The listing builds one solid part. Answer for the finished solid, in the listing's coordinates (mm). Face numbers are marked on the shaded views. A direction names the side the tool comes from. Coordinates: 2 decimals unless noted, no trailing zeros. Write each loop counter-clockwise with the first axis right and the second up, starting at its lowest first coordinate (ties: lowest second). Pieces come first, ordered by that corner, then holes.
(1) The part is cut by section D-D on x = -23. Determine the outline of the cut face in (y, z).
(2) Given P1, Ø4, axis at y = -25.5, z = -17.5, coming from the -X side; P2, Ø6, axis at x = 50.5, y = 28, coming from the -Z side; P3, Ø5.5, axis at y = 29.5, z = -18, coming from the -X side, each flat-ended and moving along its own axis, determine where each tip first touches the part or whether it passes through.
(3) The part is cut by section B-B on z = 8.5. Determine the outline of the cut face in (x, y).
(4) The part is cut by section C-C on y = 0. Determine the outline of the cut face in (x, z).
(5) The part is cut by section A-A on x = -66.5. Determine the outline of the cut face in (y, z).
(6) For a pull along X with two mould halves and no side action, classify the marked faces 1, 2 and 3 as +X half, -X half, draft (parallel to the pull), parting line (faces both ways), or undercut.
(7) Straight lines are drawn through the part: line 1 (Y direction, x = -32, z = 2); line 2 (Y direction, x = 40.5, z = -1.5); line 3 (Z direction, x = -31, y = -15). For each, find the intervals that lie inside material, in ascending order.
(8) Which of the six approach directions +Z, -Z, +X, -X, +Y, -Y give full straight-line access (tool end or side, diameter ignored) to the marked faces 4 and 5?
from build123d import *

# Parameters (mm, degrees)
F0_W      = 208
F0_H      = 50
F1_DEPTH  = 37.5
F2_R      = 32.5
F3_DEPTH  = 50.001
F4_W      = 128
F4_H      = 65
F5_DEPTH  = 45
F6_W      = 65
F6_H      = 5
F7_DEPTH  = 5
F8_W      = 10
F8_H      = 10
F9_DEPTH  = 5
F10_R     = 2
F11_DEPTH = 9.8017221311
F12_R     = 32.5
F13_W     = 125
F13_H     = 5
F14_DEPTH = 8
F16_DEPTH = 75.001


with BuildPart() as f1:
    # F0 (on Front) → F1 (new body, symmetric)
    with BuildSketch(Plane.XZ):
        Rectangle(F0_W, F0_H)
    extrude(amount=F1_DEPTH, both=True)

    # F2 (on face) → F3 (cut, through all)
    with BuildSketch(Plane.XY.offset(25)):
        with Locations((-66.5, 0)):
            Circle(F2_R)
    extrude(amount=-F3_DEPTH, mode=Mode.SUBTRACT)

    # F4 (on face) → F5 (cut)
    with BuildSketch(Plane.XY.offset(25)):
        with Locations((35, 0)):
            Rectangle(F4_W, F4_H)
    extrude(amount=-F5_DEPTH, mode=Mode.SUBTRACT)

    # F6 (on face) → F7 (cut, through all)
    with BuildSketch(Plane.YZ.offset(104)):
        with Locations((0, 22.5)):
            Rectangle(F6_W, F6_H)
    extrude(amount=-F7_DEPTH, mode=Mode.SUBTRACT)

    # F8 (on face) → F9 (join)
    with BuildSketch(Plane.XY.offset(-20)):
        with Locations((-24, 27.5)):
            Rectangle(F8_W, F8_H)
        with Locations((94, 27.5)):
            Rectangle(F8_W, F8_H)
        with Locations((-24, -27.5)):
            Rectangle(F8_W, F8_H)
        with Locations((94, -27.5)):
            Rectangle(F8_W, F8_H)
    extrude(amount=F9_DEPTH)

    # F10 (on face) → F11 (cut, through all)
    with BuildSketch(Plane.YZ.offset(-29)):
        with Locations((-15, 2)):
            Circle(F10_R)
        with Locations((15, 2)):
            Circle(F10_R)
    extrude(amount=-F11_DEPTH, mode=Mode.SUBTRACT)

    # F12
    f12_edges = [f1.edges().sort_by_distance(p)[0] for p in [
        (-104, -37.5, 0),
        (-104, 37.5, 0),
    ]]
    fillet(f12_edges, radius=F12_R)

    # F13 (on face) → F14 (join)
    with BuildSketch(Plane(origin=(0, 0, -25), x_dir=(1, 0, 0), z_dir=(0, 0, -1))):
        with Locations((41.5, 35)):
            Rectangle(F13_W, F13_H)
        with Locations((41.5, -35)):
            Rectangle(F13_W, F13_H)
    extrude(amount=F14_DEPTH)

    # F15 (on face) → F16 (cut, through all)
    with BuildSketch(Plane.XZ.offset(37.5)):
        Polygon((41.5, -25), (4, -33), (79, -33), align=None)
    extrude(amount=-F16_DEPTH, mode=Mode.SUBTRACT)


solid = f1.part
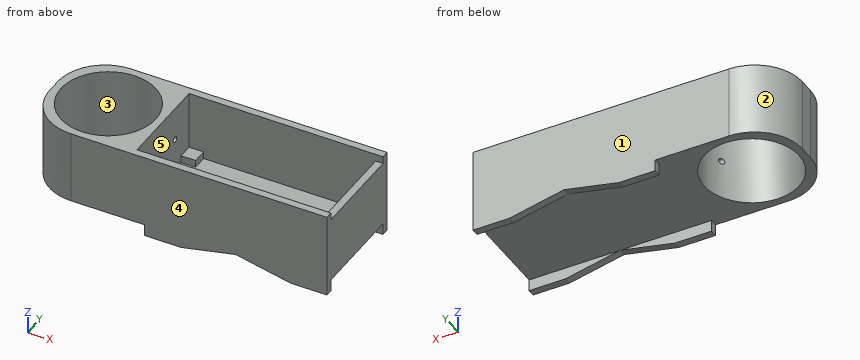
Model answer:
1. outline: (-37.5, -25) - (37.5, -25) - (37.5, 25) - (32.5, 25) - (32.5, -15) - (22.5, -15) - (22.5, -20) - (-22.5, -20) - (-22.5, -15) - (-32.5, -15) - (-32.5, 25) - (-37.5, 25) - close
2. P1: stops at x = -98.22
2. P2: stops at z = -25
2. P3: stops at x = -95.65
3. outline: (-104, -5) arc R32.5 ccw to (-71.5, -37.5) - (104, -37.5) - (104, 37.5) - (-71.5, 37.5) arc R32.5 ccw to (-104, 5) - close; hole circle Ø65 at (-66.5, 0); hole (-29, -32.5) - (99, -32.5) - (99, 32.5) - (-29, 32.5) - close
4. outline: (-104, -25) - (-99, -25) - (-99, 25) - (-104, 25) - close; (-34, -25) - (104, -25) - (104, 20) - (99, 20) - (99, -20) - (-29, -20) - (-29, 25) - (-34, 25) - close
5. outline: (-37.5, -25) - (-32.5, -25) - (-32.5, 25) - (-37.5, 25) - close; (32.5, -25) - (37.5, -25) - (37.5, 25) - (32.5, 25) - close
6. face 1: draft
6. face 2: -X half
6. face 3: undercut
7. line 1: y = -37.5 to -17, -13 to 13, 17 to 37.5
7. line 2: y = -37.5 to -32.5, 32.5 to 37.5
7. line 3: z = -25 to 0, 4 to 25
8. face 4: +Z, -Z, +X, -X, -Y
8. face 5: +Z
